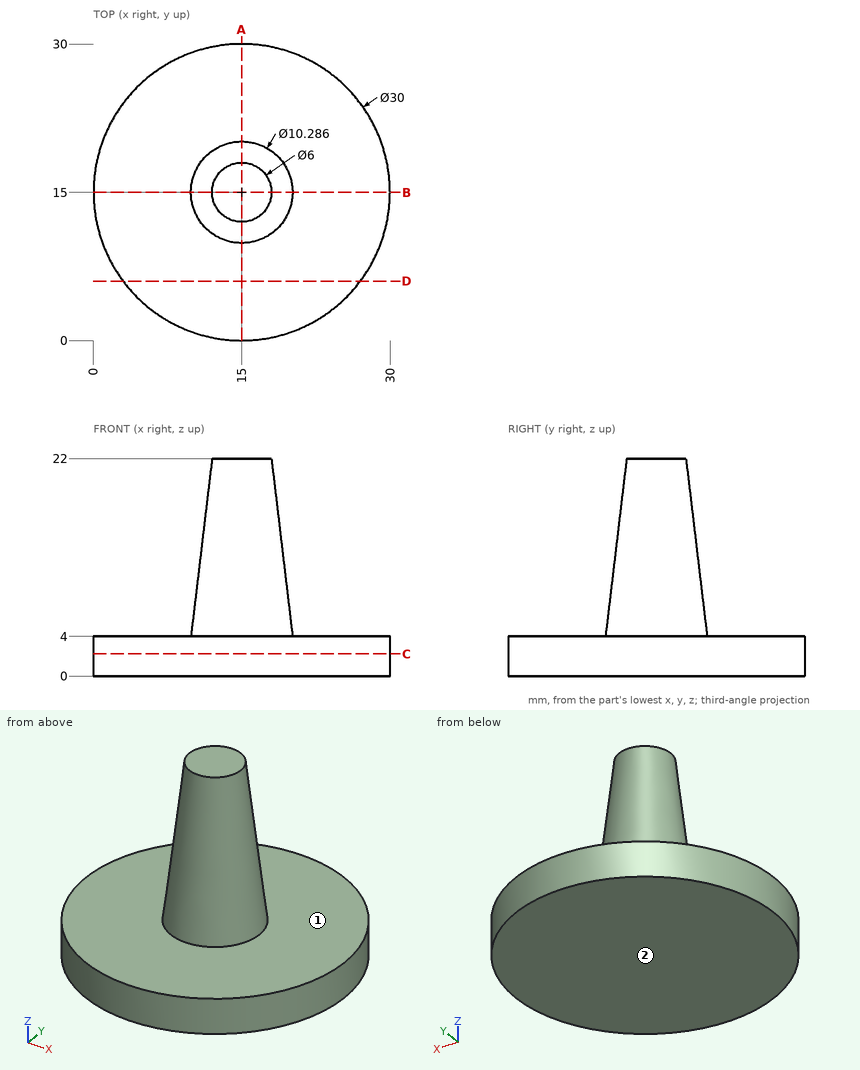
Verification items for this drawing (mm, ordinates from the low corner). A direction names the side the tool comes from. Give positions to 0.01 mm unless a question says otherwise; leave off trailing zeros. Loops run counter-clockwise (first coordinate to the right, second up) from the corner with the lowest first, then second, coordinate; pieces in that order, holes last. Notation, with made-up numbers: M 14,-8.5 L 37,-8.5 A26 ccw 37,5.5 Z; hole C -7,87.5 d8. An arc over 180 degrees is marked long. Answer as a JSON object with one key per item and string values. Group by question number.
Item 1: Sectioned sample at A-A on x = 15. Record the boundary of the cut face in (y, z).
Item 2: Access from +Z, -Z, +X, -X, +Y, -Y to the whole of each face (thin tool, end or side, straight path). Record for the marked faces 1 and 2.
Item 3: Gauge pin test, flat ends, axial feed: pin 1 (12 mm diameter, centred on y = 10, z = 9, fed in from -X) (1 decimal); pin 2 (8 mm diameter, centred on x = 13.5, z = 5, fed in from -Y); pin 3 (5 mm diameter, centred on x = 10.5, z = 12, fed in from +Y); pin 4 (2 mm diameter, centred on x = 8.5, z = 7, fed in from +Y). Record the tip position at first contact, or that the pin passes through.
Item 4: Material ranges on L1, parallel to Z at x = 27.25, y = 8.75; L2, parallel to X at y = 24, z = 3.75; L3, parallel to Y at x = 17, z = 3, recorded low to high.
Item 5: Sectioned sample at C-C on z = 2.25. Record the boundary of the cut face in (x, y).
Item 6: Sectioned sample at D-D on y = 6. Record the boundary of the cut face in (x, z).
Findings below:
{
 "1": {"outline": "M 0,0 L 30,0 L 30,4 L 20.14,4 L 18,22 L 12,22 L 9.86,4 L 0,4 Z"},
 "2": {"face 1": "+Z", "face 2": "-Z, +X, -X, +Y, -Y"},
 "3": {"pin 1": "x = 0.1", "pin 2": "y = 0", "pin 3": "y = 18.72", "pin 4": "through"},
 "4": {"L1": "0 to 4", "L2": "3 to 27", "L3": "0.13 to 29.87"},
 "5": {"outline": "C 15,15 d30"},
 "6": {"outline": "M 3,0 L 27,0 L 27,4 L 3,4 Z"}
}
